Geometry check sheet. Reference: the model listing, model coordinates, mm. A direction names the side the tool comes from. Give positions to 0.01 mm unless a question says otherwise; leave off trailing zeros. Write each loop counter-clockwise with the first axis right and the second up, starting at its lowest first coordinate (ties: lowest second). Pieces come first, ordered by that corner, then holes. Notation, with made-up numbers: (10.25, 34.25) - (15.25, 34.25) arc R27 ccw to (15.25, 50.25) - close; hole circle Ø1 at (20, -16.5). An arc over 180 degrees is marked (long way). Write item = value, one per line. Start each with the question number.
(1) Section check B-B, the plane x = 0. Enter the section's corners in (y, z).
(2) Draft check along Y on faces 4 (the cylindrical face through (-29.04, 137.24, -49.94)), 5 (the flat face through (-1, 0, -2)), 6 (the cylindrical face through (-29.45, 91.08, -59.49)). Enter one of: pulls with the +Y half, pulls with the -Y half, needs draft (parallel to the pull), parting line crosses it, or undercut.
(3) Depth check by flat-ended pin: pin 1 Ø6 at (x, z) = (-19.5, 46) entering from -Y; pin 2 Ø9 at (x, y) = (-26.5, 89.2) entering from +Z. Enter the tip coordinate at first touch or a pass-through.
(4) Access from +Z, -Z, +X, -X, +Y, -Y to the whole of each face (thin tool, end or side, straight path). Record for faces 1 (the cylindrical face through (-0.521, 0.986, 27.466)), 2 (the flat face through (-1, 136.25, -1)), 3 (the cylindrical face through (27.96, 137.24, -49.94)).
(5) Section check A-A, the plane z = 50.5. Enter the section's corners in (x, y), plus the area to 3 significant figures.
(6) Thickness scan on L1, parallel to Z at x = 28.5, y = 136.7; L2, parallel to Y at x = -30, z = 26; L3, parallel to Z at x = -28, y = 137. Record the ranges inside material, lowest first.
(7) Section check C-C, the plane y = 89.2. Enter the section's corners in (x, z), plus the area to 3 significant figures.
(8) Section check D-D, the plane z = 23.5. Enter the section's corners in (x, y).
```python
from build123d import *

# Parameters (mm, degrees)
ESBO_O1_W                = 75
ESBO_O1_H                = 117
RESSALTO_EXTRUS_O1_DEPTH = 2
ESBO_O2_W                = 75
ESBO_O2_H                = 2
RESSALTO_EXTRUS_O2_DEPTH = 136.25
ESBO_O3_W                = 75
ESBO_O3_H                = 119
RESSALTO_EXTRUS_O3_DEPTH = 2
ESBO_O4_R                = 2.5
CORTE_EXTRUS_O1_DEPTH    = 139.25
ESBO_O5_R                = 7.5
CORTE_EXTRUS_O2_DEPTH    = 10
CORTE_EXTRUS_O3_DEPTH    = 10
ESBO_O7_R                = 4
CORTE_EXTRUS_O4_DEPTH    = 10


with BuildPart() as part:
    # Esboço1 → Ressalto-extrusão1 (new body)
    with BuildSketch(Plane(origin=(0, 0, 0), x_dir=(1, 0, 0), z_dir=(0, 1, 0))):
        Rectangle(ESBO_O1_W, ESBO_O1_H)
    extrude(amount=RESSALTO_EXTRUS_O1_DEPTH)

    # Esboço2 → Ressalto-extrusão2 (add)
    with BuildSketch(Plane(origin=(0, 0, 0), x_dir=(1, 0, 0), z_dir=(0, 1, 0))):
        with Locations((0, 59.5)):
            Rectangle(ESBO_O2_W, ESBO_O2_H)
    extrude(amount=RESSALTO_EXTRUS_O2_DEPTH)

    # Esboço3 → Ressalto-extrusão3 (add)
    with BuildSketch(Plane(origin=(0, 136.25, 0), x_dir=(1, 0, 0), z_dir=(0, 1, 0))):
        with Locations((0, 1)):
            Rectangle(ESBO_O3_W, ESBO_O3_H)
    extrude(amount=RESSALTO_EXTRUS_O3_DEPTH)

    # Esboço4 → Corte-extrusão1 (cut, through all)
    with BuildSketch(Plane.XZ):
        with Locations((28.5, -47.5)):
            Circle(ESBO_O4_R)
        with Locations((-28.5, -47.5)):
            Circle(ESBO_O4_R)
        with Locations((28.5, 50.5)):
            Circle(ESBO_O4_R)
        with Locations((-28.5, 50.5)):
            Circle(ESBO_O4_R)
    extrude(amount=-CORTE_EXTRUS_O1_DEPTH, mode=Mode.SUBTRACT)

    # Esboço5 → Corte-extrusão2 (cut)
    with BuildSketch(Plane(origin=(0, 0, -60.5), x_dir=(-1, 0, 0), z_dir=(0, 0, -1))):
        with Locations((0, 89.2)):
            Circle(ESBO_O5_R)
    extrude(amount=-CORTE_EXTRUS_O2_DEPTH, mode=Mode.SUBTRACT)

    # Esboço6 → Corte-extrusão3 (cut)
    with BuildSketch(Plane.XY.offset(-58.5)):
        with BuildLine():
            ThreePointArc((26.5, 85.7), (30, 89.2), (26.5, 92.7))
            ThreePointArc((26.5, 92.7), (23, 89.2), (26.5, 85.7))
        make_face()
        with BuildLine():
            ThreePointArc((-26.5, 85.7), (-23, 89.2), (-26.5, 92.7))
            ThreePointArc((-26.5, 92.7), (-30, 89.2), (-26.5, 85.7))
        make_face()
    extrude(amount=-CORTE_EXTRUS_O3_DEPTH, mode=Mode.SUBTRACT)

    # Esboço7 → Corte-extrusão4 (cut)
    with BuildSketch(Plane.XZ):
        with Locations((0, -38.5)):
            Circle(ESBO_O7_R)
        with Locations((0, 23.5)):
            Circle(ESBO_O7_R)
    extrude(amount=-CORTE_EXTRUS_O4_DEPTH, mode=Mode.SUBTRACT)


solid = part.part
```
Model answer:
q1.outline = (0, -60.5) - (81.7, -60.5) - (81.7, -58.5) - (2, -58.5) - (2, -42.5) - (0, -42.5) - close; (0, -34.5) - (2, -34.5) - (2, 19.5) - (0, 19.5) - close; (0, 27.5) - (2, 27.5) - (2, 58.5) - (0, 58.5) - close; (96.7, -60.5) - (138.25, -60.5) - (138.25, 58.5) - (136.25, 58.5) - (136.25, -58.5) - (96.7, -58.5) - close
q2.face_4 = needs draft
q2.face_5 = pulls with the -Y half
q2.face_6 = undercut
q3.pin_1 = 0
q3.pin_2 = -58.5
q4.face_1 = -Y
q4.face_2 = +Z, +X, -X
q4.face_3 = +Y, -Y
q5.outline = (-37.5, 0) - (-31, 0) - (-31, 2) - (-37.5, 2) - close; (-37.5, 136.25) - (-31, 136.25) - (-31, 138.25) - (-37.5, 138.25) - close; (-26, 0) - (26, 0) - (26, 2) - (-26, 2) - close; (-26, 136.25) - (26, 136.25) - (26, 138.25) - (-26, 138.25) - close; (31, 0) - (37.5, 0) - (37.5, 2) - (31, 2) - close; (31, 136.25) - (37.5, 136.25) - (37.5, 138.25) - (31, 138.25) - close
q5.area = 260 mm²
q6.L1 = -60.5 to -50, -45 to 48, 53 to 58.5
q6.L2 = 0 to 2, 136.25 to 138.25
q6.L3 = -60.5 to -49.95, -45.05 to 48.05, 52.95 to 58.5
q7.outline = (-37.5, -60.5) - (-30, -60.5) - (-30, -58.5) - (-37.5, -58.5) - close; (-23, -60.5) - (-7.5, -60.5) - (-7.5, -58.5) - (-23, -58.5) - close; (7.5, -60.5) - (23, -60.5) - (23, -58.5) - (7.5, -58.5) - close; (30, -60.5) - (37.5, -60.5) - (37.5, -58.5) - (30, -58.5) - close
q7.area = 92.0 mm²
q8.outline = (-37.5, 0) - (-4, 0) - (-4, 2) - (-37.5, 2) - close; (-37.5, 136.25) - (37.5, 136.25) - (37.5, 138.25) - (-37.5, 138.25) - close; (4, 0) - (37.5, 0) - (37.5, 2) - (4, 2) - close
